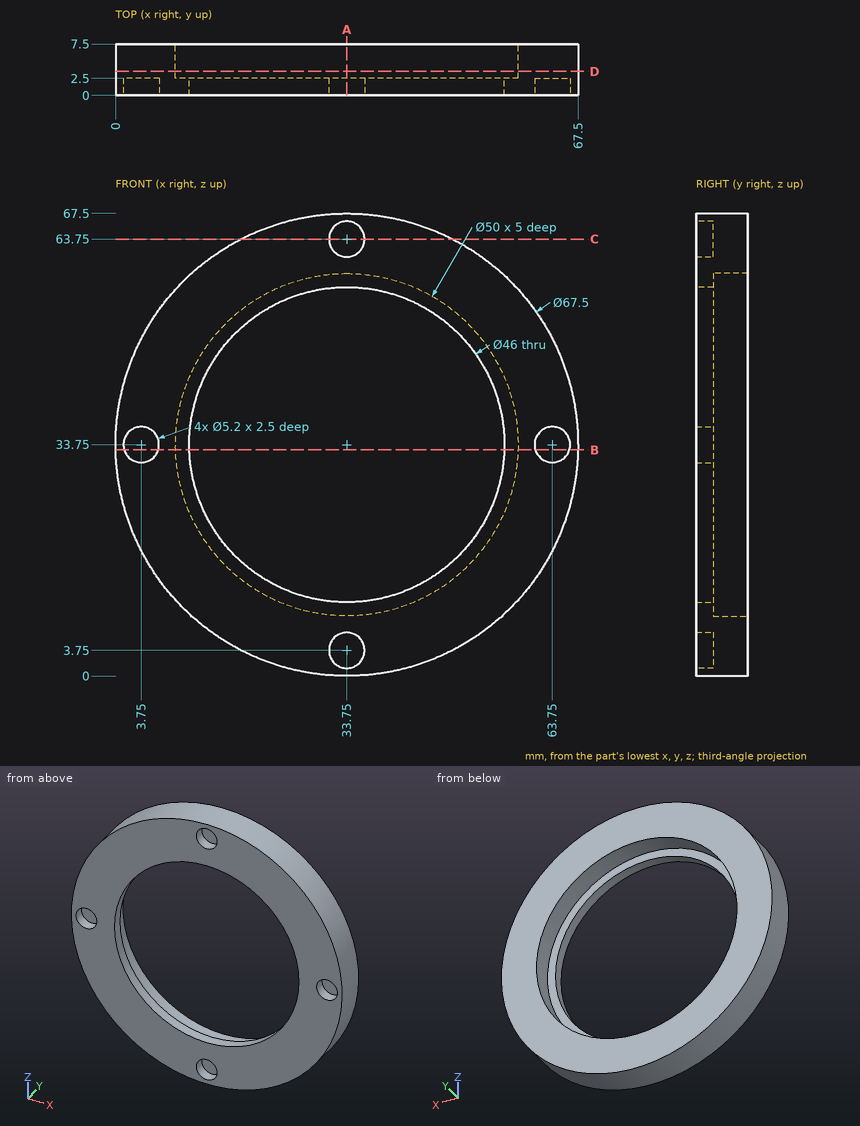
The figure shows three views and two pictorial views of one solid part (mm, origin at its lowest corner). Answer the questions. Give positions to 0.01 mm unless a question says otherwise; leave off trailing zeros. Loops run counter-clockwise (first coordinate to the right, second up) from the corner with the lowest first, then second, coordinate; pieces in that order, holes last. Notation, with made-up numbers: (19, -6) - (40, -6) arc R32 cw to (40, 28) - close; hole circle Ø7 at (-33, -22.75). An arc over 180 degrees is marked (long way). Answer in a Markdown table with one row per item.
(1) Section D-D (y = 3.5) is taken. Give the vertices of the cut face in (x, z).
Results list:
| item | result |
|---|---|
| outline | circle Ø67.5 at (33.75, 33.75); hole circle Ø50 at (33.75, 33.75) |
(2) Section C-C (z = 63.75) is taken. Give the vertices of the cut face in (x, y).
Results list:
| item | result |
|---|---|
| outline | (18.29, 0) - (31.15, 0) - (31.15, 2.5) - (36.35, 2.5) - (36.35, 0) - (49.21, 0) - (49.21, 7.5) - (18.29, 7.5) - close |
(3) Consider L1, parallel to X at y = 0.75, z = 33.75; L2, parallel to X at y = 3.5, z = 33.75; L3, parallel to Z at x = 36, y = 1.25. Determine where each line is inside the solid, lowest interval first. Write a range as [from, to].
Results list:
| item | result |
|---|---|
| L1 | x = [0, 1.15], [6.35, 10.75], [56.75, 61.15], [66.35, 67.5] |
| L2 | x = [0, 8.75], [58.75, 67.5] |
| L3 | z = [0.08, 2.45], [5.05, 10.86], [56.64, 62.45], [65.05, 67.42] |
(4) Section A-A (x = 33.75) is taken. Give the vertices of the cut face in (y, z), and give its area (3 significant figures).
Results list:
| item | result |
|---|---|
| outline | (0, 0) - (7.5, 0) - (7.5, 8.75) - (2.5, 8.75) - (2.5, 10.75) - (0, 10.75) - (0, 6.35) - (2.5, 6.35) - (2.5, 1.15) - (0, 1.15) - close; (0, 56.75) - (2.5, 56.75) - (2.5, 58.75) - (7.5, 58.75) - (7.5, 67.5) - (0, 67.5) - (0, 66.35) - (2.5, 66.35) - (2.5, 61.15) - (0, 61.15) - close |
| area | 115 mm² |
(5) Section B-B (z = 33) is taken. Give the vertices of the cut face in (x, y), and give its area (3 significant figures).
Results list:
| item | result |
|---|---|
| outline | (0.01, 0) - (1.26, 0) - (1.26, 2.5) - (6.24, 2.5) - (6.24, 0) - (10.76, 0) - (10.76, 2.5) - (8.76, 2.5) - (8.76, 7.5) - (0.01, 7.5) - close; (56.74, 0) - (61.26, 0) - (61.26, 2.5) - (66.24, 2.5) - (66.24, 0) - (67.49, 0) - (67.49, 7.5) - (58.74, 7.5) - (58.74, 2.5) - (56.74, 2.5) - close |
| area | 116 mm² |
(6) Flat-ended cylindrical pins translate along their axes: pin 1 Ø2.5 at (x, z) = (4, 33) entering from -Y; pin 2 Ø5.5 at (x, z) = (64.5, 33.5) entering from -Y; pin 3 Ø1 at (y, z) = (6.5, 27.5) entering from -X; pin 4 Ø10 at (x, z) = (15, 30) entering from +Y. Find the tip coordinate at first contact, or state that the pin passes through.
Results list:
| item | result |
|---|---|
| pin 1 | stops at y = 2.5 |
| pin 2 | stops at y = 0 |
| pin 3 | stops at x = 0.49 |
| pin 4 | stops at y = 2.5 |
